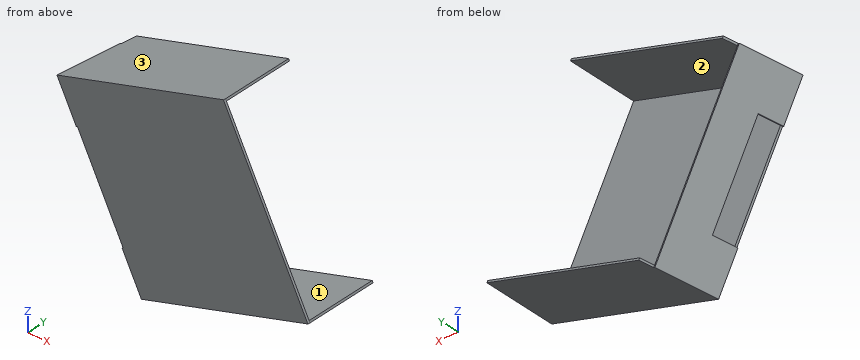
from build123d import *

# Parameters (mm, degrees)
BOSS_EXTRUDE1_DEPTH = 609.6
CUT_EXTRUDE1_DEPTH  = 596.9
CUT_EXTRUDE2_START  = -6.35
CUT_EXTRUDE2_DEPTH  = 6.35


with BuildPart() as part:
    # Sketch1 → Boss-Extrude1 (new body)
    with BuildSketch(Plane(origin=(2274.798526179, 0, -4526.609622936), x_dir=(0.8935178411679832, 0, 0.44902769125579206), z_dir=(-0.44902769125579206, 0, 0.8935178411679832))):
        Polygon((-4499.407931927, 647.178189885), (-4499.091966051, 887.542246672), (-5297.754801193, 1148.204732428), (-5311.546165746, 1105.948362922), (-5317.582789961, 1107.918557858), (-5376.688638045, 926.819831407), (-4501.378126863, 641.14156567), align=None)
    extrude(amount=-BOSS_EXTRUDE1_DEPTH)

    # Sketch2 → Cut-Extrude1 (cut)
    with BuildSketch(Plane(origin=(2277.649852018, 0, -4532.283461227), x_dir=(-0.8935178411679832, 0, -0.44902769125579206), z_dir=(0.44902769125579206, 0, -0.8935178411679832))):
        Polygon((5297.754801193, 1148.204732428), (4977.813717796, 1043.784400813), (4499.091966051, 887.542246672), (4499.407931927, 647.178189885), (5368.681818894, 930.886260686), align=None)
    extrude(amount=CUT_EXTRUDE1_DEPTH, mode=Mode.SUBTRACT)

    # Sketch3 → Cut-Extrude2 (cut)
    with BuildSketch(Plane(origin=(-4585.952542808, 1675.102491314, -2304.620666347), x_dir=(-0.40095713367550895, 0.14645687831706847, 0.9043139718860588), z_dir=(-0.8494222734757242, 0.31026691907399934, -0.4268679424033393)).offset(CUT_EXTRUDE2_START)):
        Polygon((-5579.388539548, 150.427587067), (-5591.127897041, 75.137298944), (-5264.869981841, 24.266749807), (-5253.130624348, 99.55703793), align=None)
    extrude(amount=CUT_EXTRUDE2_DEPTH, mode=Mode.SUBTRACT)


solid = part.part
Model file for the job. Use its own axes, mm. Face numbers are marked on the shaded views. Give positions to 0.01 mm unless a question says otherwise; leave off trailing zeros. Loops run counter-clockwise (first coordinate to the right, second up) from the corner with the lowest first, then second, coordinate; pieces in that order, holes last. Notation, with made-up numbers: (50, -35.75) -> (99, -35.75) arc R21 ccw to (99, -14.75) -> close; hole circle Ø8 at (-20.75, 17.25). An arc over 180 degrees is marked (long way). Use a Markdown table: item, result. Add a question column.
(1) Mould opens along X. For the marked faces 1, 2 and 3 say: +X half, -X half, draft (parallel to the pull), parting line (faces both ways), or undercut.
(2) Slice it at C-C on x = -1782.5. List the corners of the cut face in (y, z), and give its area (3 significant figures).
(3) Slice it at A-A on z = -7218.5. List the corners of the cut face in (x, y), and give its area (3 significant figures).
(4) Slice it at D-D on y = 1090.5. List the corners of the cut face in (x, z).
(5) Wall check: line 1 along Z through (x, y) = (-2094, 1012); line 2 along Z through (x, y) = (-1899.5, 1009.5); line 3 along Y through (x, z) = (-1637, -6941.5). Give the ranges that are in metal, low to high.
(6) Drop flat-ended pins along their axis: pin 1 Ø12 at (x, z) = (-2198, -6773.5) entering from +Y; pin 2 Ø1.5 at (x, y) = (-2082.5, 831) entering from +Z; pin 3 Ø8 at (y, z) = (761, -6655) entering from +X. Give the stop position or say it passes through.
(7) Slice it at B-B on y = 974. List the corners of the cut face in (x, z), and give its area (3 significant figures).
Filled sheet:
| question | item | result |
|---|---|---|
| 1 | face 1 | undercut |
| 1 | face 2 | +X half |
| 1 | face 3 | -X half |
| 2 | outline | (654.01, -6565.56) -> (754, -7247.81) -> (1001.14, -7247.81) -> (1000.1, -7240.7) -> (759.63, -7240.7) -> (661.73, -6572.67) -> (902.2, -6572.67) -> (901.16, -6565.56) -> close |
| 2 | area | 7,980 mm2 |
| 3 | outline | (-2383.1, 924.85) -> (-1724.18, 732.69) -> (-1724.18, 979.84) -> (-1738.32, 983.96) -> (-1738.32, 743.5) -> (-2380.9, 930.89) -> close; (-2363.4, 999.26) -> (-2356.64, 997.29) -> (-2316.95, 1105.95) -> (-2323.71, 1107.92) -> close |
| 3 | area | 8,610 mm2 |
| 4 | outline | (-2481.64, -6916.9) -> (-2207.91, -7461.59) -> (-2027.13, -7370.75) -> (-2029.98, -7365.07) -> (-2204.79, -7452.92) -> (-2472.82, -6919.58) -> (-2298.01, -6831.73) -> (-2300.86, -6826.06) -> close |
| 5 | line 1 | -7404.35 to -7397.24, -6729.21 to -6722.1 |
| 5 | line 2 | -7306.61 to -7299.5 |
| 5 | line 3 | 666.68 to 673.36 |
| 6 | pin 1 | y = 1054.74 |
| 6 | pin 2 | z = -6715.95 |
| 6 | pin 3 | x = -1938.37 |
| 7 | outline | (-2515.61, -6933.98) -> (-2452.88, -7058.8) -> (-2446.91, -7055.8) -> (-2506.79, -6936.65) -> (-1979.07, -6671.45) -> (-1981.92, -6665.78) -> close; (-2304.61, -7353.84) -> (-2241.88, -7478.67) -> (-1708.19, -7210.46) -> (-1711.04, -7204.79) -> (-2238.77, -7469.99) -> (-2298.64, -7350.84) -> close |
| 7 | area | 9,370 mm2 |
